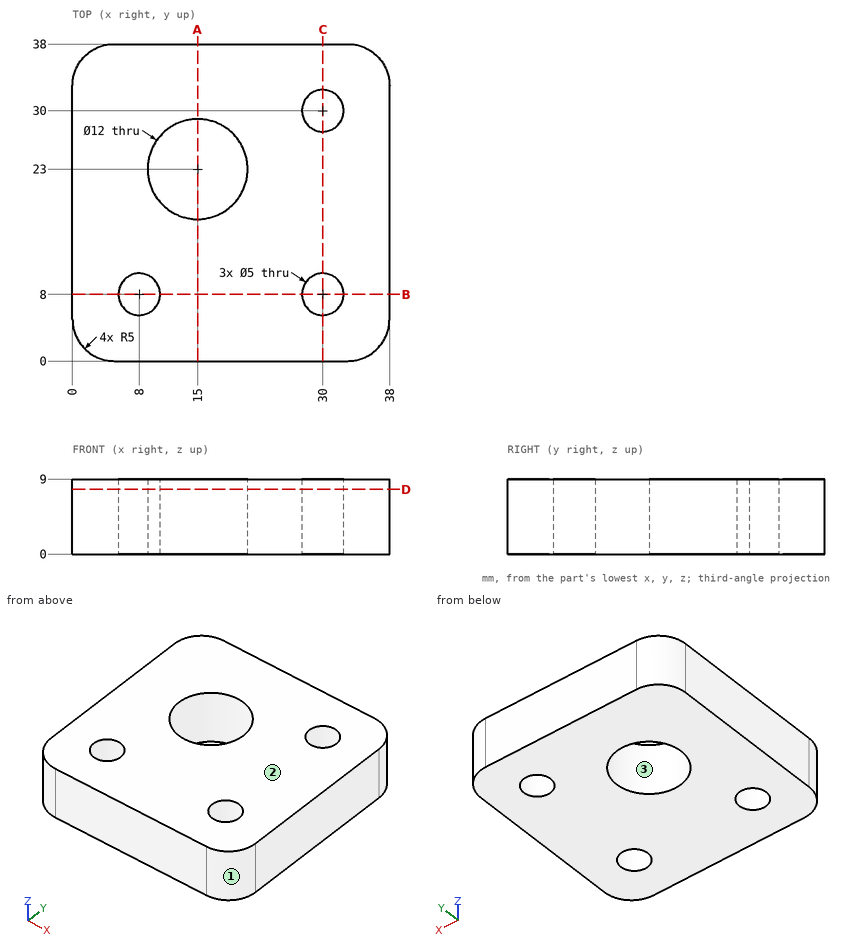
The drawing under review shows one solid part. Ordinate dimensions are in mm from its lowest x, y, z. Give positions to 0.01 mm unless a question says otherwise; leave off trailing zeros. Order: outer loops, then holes, each group sorted by start corner. A loop starts at its lowest first (then second) coordinate and runs counter-clockwise, first axis right, second up. Notation, with made-up numbers: (3.25, -34.75) -> (12.25, -34.75) arc R25 ccw to (12.25, -12.75) -> close; hole circle Ø10 at (2, 8.25). An arc over 180 degrees is marked (long way). Write item = value, one per line. Start each with the question number.
(1) We need section D-D on z = 7.75. Write out the cut boundary in (x, y), plus the area to 3 significant figures.
(2) To check wall thickness, follow line 1 along Y through (x, z) = (30, 7); line 2 along X through (y, z) = (7, 3.25); line 3 along X through (y, z) = (8.5, 7.25). State the ranges of each line that lie inside material, in increasing order.
(3) We need section A-A on x = 15. Write out the cut boundary in (y, z).
(4) For pin 1 (4 mm diameter, centred on x = 30, y = 8, fed in from +Z), flat-tipped, find the tip position at first contact; note if it passes through.
(5) Mouldability with a two-part tool opening along X and no side actions: class the marked faces 1, 2 and 3 as +X half, -X half, draft (parallel to the pull), parting line (faces both ways), or undercut.
(6) We need section B-B on y = 8. Write out the cut boundary in (x, z).
Numbers:
q1.outline = (0, 5) arc R5 ccw to (5, 0) -> (33, 0) arc R5 ccw to (38, 5) -> (38, 33) arc R5 ccw to (33, 38) -> (5, 38) arc R5 ccw to (0, 33) -> close; hole circle Ø5 at (8, 8); hole circle Ø12 at (15, 23); hole circle Ø5 at (30, 8); hole circle Ø5 at (30, 30)
q1.area = 1,250 mm^2
q2.line_1 = 0 to 5.5, 10.5 to 27.5, 32.5 to 38
q2.line_2 = 0 to 5.71, 10.29 to 27.71, 32.29 to 38
q2.line_3 = 0 to 5.55, 10.45 to 27.55, 32.45 to 38
q3.outline = (0, 0) -> (17, 0) -> (17, 9) -> (0, 9) -> close; (29, 0) -> (38, 0) -> (38, 9) -> (29, 9) -> close
q4.pin_1 = through
q5.face_1 = +X half
q5.face_2 = draft
q5.face_3 = undercut
q6.outline = (0, 0) -> (5.5, 0) -> (5.5, 9) -> (0, 9) -> close; (10.5, 0) -> (27.5, 0) -> (27.5, 9) -> (10.5, 9) -> close; (32.5, 0) -> (38, 0) -> (38, 9) -> (32.5, 9) -> close
